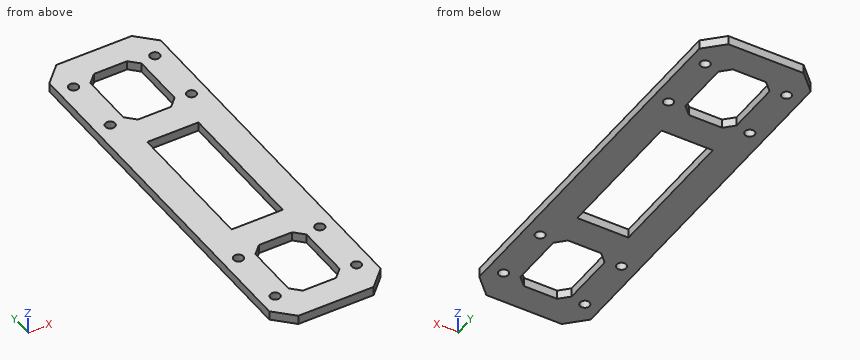
```python
from build123d import *

# Parameters (mm, degrees)
SKETCH_1_W          = 37
SKETCH_1_H          = 120
SKETCH_1_R          = 1.6
EXTRUDE_1_DEPTH     = 3
SKETCH_2_W          = 17
SKETCH_2_H          = 24
CUT_EXTRUDE_1_DEPTH = 126.610509114
SKETCH_3_W          = 37
SKETCH_3_H          = 6
EXTRUDE_2_DEPTH     = 3
CHAMFER_1_SIZE      = 6
CHAMFER_2_SIZE      = 3
SKETCH_4_W          = 17
SKETCH_4_H          = 46
CUT_EXTRUDE_2_DEPTH = 10


with BuildPart() as part:
    # ｽｹｯﾁ1 → ﾎﾞｽ - 押し出し1 (new body)
    with BuildSketch(Plane.XY):
        with Locations((18.5, 60)):
            Rectangle(SKETCH_1_W, SKETCH_1_H)
        with Locations((5, 115)):
            Circle(SKETCH_1_R, mode=Mode.SUBTRACT)
        with Locations((32, 115)):
            Circle(SKETCH_1_R, mode=Mode.SUBTRACT)
        with Locations((5, 95)):
            Circle(SKETCH_1_R, mode=Mode.SUBTRACT)
        with Locations((32, 95)):
            Circle(SKETCH_1_R, mode=Mode.SUBTRACT)
        with Locations((5, 25)):
            Circle(SKETCH_1_R, mode=Mode.SUBTRACT)
        with Locations((32, 25)):
            Circle(SKETCH_1_R, mode=Mode.SUBTRACT)
        with Locations((5, 5)):
            Circle(SKETCH_1_R, mode=Mode.SUBTRACT)
        with Locations((32, 5)):
            Circle(SKETCH_1_R, mode=Mode.SUBTRACT)
    extrude(amount=EXTRUDE_1_DEPTH)

    # ｽｹｯﾁ2 → ｶｯﾄ - 押し出し1 (cut, through all)
    with BuildSketch(Plane.XY.offset(3)):
        with Locations((18.5, 105)):
            Rectangle(SKETCH_2_W, SKETCH_2_H)
        with Locations((18.5, 15)):
            Rectangle(SKETCH_2_W, SKETCH_2_H)
    extrude(amount=-CUT_EXTRUDE_1_DEPTH, mode=Mode.SUBTRACT)

    # ｽｹｯﾁ3 → ﾎﾞｽ - 押し出し2 (add)
    with BuildSketch(Plane.XY.offset(3)):
        with Locations((18.5, 123)):
            Rectangle(SKETCH_3_W, SKETCH_3_H)
        with Locations((18.5, -3)):
            Rectangle(SKETCH_3_W, SKETCH_3_H)
    extrude(amount=-EXTRUDE_2_DEPTH)

    # 面取り1
    chamfer_1_edges = [part.edges().sort_by_distance(p)[0] for p in [
        (0, 126, 1.5),
        (37, 126, 1.5),
        (0, -6, 1.5),
        (37, -6, 1.5),
    ]]
    chamfer(chamfer_1_edges, length=CHAMFER_1_SIZE)

    # 面取り2
    chamfer_2_edges = [part.edges().sort_by_distance(p)[0] for p in [
        (10, 93, 1.5),
        (10, 117, 1.5),
        (27, 117, 1.5),
        (27, 93, 1.5),
        (10, 3, 1.5),
        (10, 27, 1.5),
        (27, 27, 1.5),
        (27, 3, 1.5),
    ]]
    chamfer(chamfer_2_edges, length=CHAMFER_2_SIZE)

    # ｽｹｯﾁ4 → ｶｯﾄ - 押し出し2 (cut)
    with BuildSketch(Plane.XY.offset(3)):
        with Locations((18.5, 60)):
            Rectangle(SKETCH_4_W, SKETCH_4_H)
    extrude(amount=-CUT_EXTRUDE_2_DEPTH, mode=Mode.SUBTRACT)


solid = part.part
```
Source: CAD feature listing. Evaluate the final solid. Frame: model axes, mm. Round coordinates to 2 decimals unless told otherwise and drop trailing zeros. Loops run counter-clockwise (first coordinate to the right, second up) from the corner with the lowest first, then second, coordinate; pieces in that order, holes last. Notation, with made-up numbers: M 39.25,15.5 L 94.25,15.5 A19 cw 94.25,27.5 Z; hole C 65.25,68.5 d10. An arc over 180 degrees is marked long. Use a Markdown table: item, result. Add a question column.
1. Cut plane A-A, the plane x = 18.5. Output: boundary loops of the cut face in (y, z), and give its area (3 significant figures).
2. Ray query, line 1 along X through (y, z) = (104.5, 1); line 2 along Y through (x, z) = (15.5, 0.3); line 3 along Y through (x, z) = (4.5, 1.05). Return the intervals inside material, ascending. Write a range as [from, to].
3. Contact query for flat-ended pins moving along their axis: pin 1 (1.9 mm diameter, centred on x = 32, y = 95, fed in from -Z) (3 decimals); pin 2 (5 mm diameter, centred on x = 5, y = 25, fed in from -Z). Output: stop coordinate, or through.
4. Cut plane B-B, the plane y = 57.5. Output: boundary loops of the cut face in (x, z), and give its area (3 significant figures).
5. Cut plane C-C, the plane z = 0.65. State how many separate pieces and enclosed holes the cut face has, and give its area (3 significant figures).
Solution:
| question | item | result |
|---|---|---|
| 1 | outline | M -6,0 L 3,0 L 3,3 L -6,3 Z; M 27,0 L 37,0 L 37,3 L 27,3 Z; M 83,0 L 93,0 L 93,3 L 83,3 Z; M 117,0 L 126,0 L 126,3 L 117,3 Z |
| 1 | area | 114 mm2 |
| 2 | line 1 | x = [0, 10], [27, 37] |
| 2 | line 2 | y = [-6, 3], [27, 37], [83, 93], [117, 126] |
| 2 | line 3 | y = [-4.5, 3.48], [6.52, 23.48], [26.52, 93.48], [96.52, 113.48], [116.52, 124.5] |
| 3 | pin 1 | passes through |
| 3 | pin 2 | stops at z = 0 |
| 4 | outline | M 0,0 L 10,0 L 10,3 L 0,3 Z; M 27,0 L 37,0 L 37,3 L 27,3 Z |
| 4 | area | 60.0 mm2 |
| 5 | separate pieces | 1 |
| 5 | enclosed holes | 11 |
| 5 | area | 3,190 mm2 |
